For this review, take the finished solid that the model builds, in its own axes (mm). Face numbers are marked on the shaded views. Coordinates: 2 decimals unless noted, no trailing zeros. Order: outer loops, then holes, each group sorted by start corner. A loop starts at its lowest first (then second) coordinate and runs counter-clockwise, first axis right, second up. Notation, with made-up numbers: (10, 67.25) -> (57, 67.25) arc R26 cw to (57, 98.25) -> close; hole circle Ø6 at (66.25, 15). An arc over 180 degrees is marked (long way). Answer as a JSON object with one key per item and string values. Group by question number.
1) Add section D-D, the plane z = 9.5. Write out the cut boundary in (x, y), then the cut area to 3 significant figures.
2) Wall thickness on L1, parallel to X at y = 5, z = 5; L2, parallel to X at y = -17, z = 2; L3, parallel to Y at x = -13, z = 2: over which ranges is each line inside the solid? List them lowest first.
3) Add section A-A, the plane y = 0. Write out the cut boundary in (x, z).
4) Add section C-C, the plane y = -21. Write out the cut boundary in (x, z), then the cut area to 3 significant figures.
5) For pin 1 (18.5 mm diameter, centred on x = -12.51, y = 13.19, fed in from +Z); pin 2 (8 mm diameter, centred on x = -23, z = 7.5, fed in from -Y); pin 3 (12 mm diameter, centred on x = -12.5, y = -20.5, fed in from +Z); pin 4 (1 mm diameter, centred on x = 21, z = 3.5, fed in from +Y), all flat-tipped, find the tip position at first contact; note any pin that passes through.
6) Draft analysis for pull direction X (two halves, no side actions). For the marked faces 1, 2, 3 and 4, state which applies: +X half, -X half, draft (parallel to the pull), parting line (faces both ways), or undercut.
7) Add section B-B, the plane x = 13. Write out the cut boundary in (y, z).
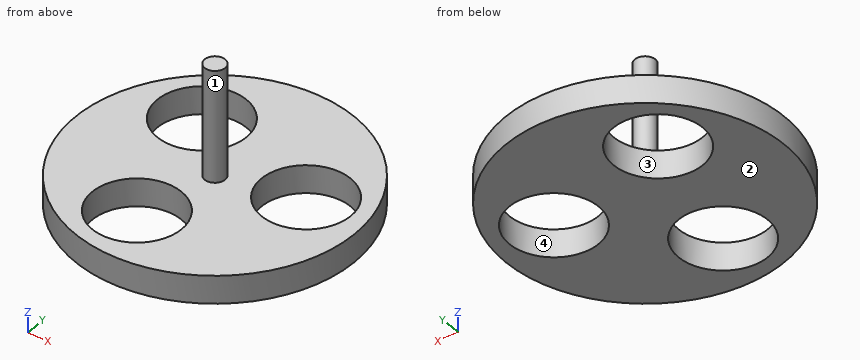
from build123d import *

# Parameters (mm, degrees)
F0_R     = 31.75
F2_DEPTH = 6.35
F1_R     = 10.16
F3_DEPTH = 25.4
F4_R     = 2.336661
F5_DEPTH = 25.4


with BuildPart() as f2:
    # F0 (on Top) → F2 (new body)
    with BuildSketch(Plane.XY):
        Circle(F0_R)
    extrude(amount=F2_DEPTH)

    # F1 (on face) → F3 (cut)
    with BuildSketch(Plane.XY):
        with Locations((-5.168118, -17.430304)):
            Circle(F1_R)
        with Locations((17.679145, 4.23943)):
            Circle(F1_R)
        with Locations((-12.511027, 13.190874)):
            Circle(F1_R)
    extrude(amount=F3_DEPTH, mode=Mode.SUBTRACT)

    # F4 (on face) → F5 (join)
    with BuildSketch(Plane.XY.offset(6.35)):
        Circle(F4_R)
    extrude(amount=F5_DEPTH)


solid = f2.part
Output values:
{
 "1": {"outline": "circle Ø4.67 at (0, 0)", "area": "17.2 mm²"},
 "2": {"L1": "x = -31.35 to -18.52, -6.5 to 7.55, 27.81 to 31.35", "L2": "x = -26.82 to -15.32, 4.98 to 26.82", "L3": "y = -28.97 to -23.9, -10.96 to 3.04, 23.34 to 28.97"},
 "3": {"outline": "(-31.75, 0) -> (8.45, 0) -> (8.45, 6.35) -> (2.34, 6.35) -> (2.34, 31.75) -> (-2.34, 31.75) -> (-2.34, 6.35) -> (-31.75, 6.35) -> close; (26.91, 0) -> (31.75, 0) -> (31.75, 6.35) -> (26.91, 6.35) -> close"},
 "4": {"outline": "(-23.81, 0) -> (-14.68, 0) -> (-14.68, 6.35) -> (-23.81, 6.35) -> close; (4.34, 0) -> (23.81, 0) -> (23.81, 6.35) -> (4.34, 6.35) -> close", "area": "182 mm²"},
 "5": {"pin 1": "passes through", "pin 2": "stops at y = -25.31", "pin 3": "stops at z = 6.35", "pin 4": "stops at y = 24.24"},
 "6": {"face 1": "parting line", "face 2": "draft", "face 3": "undercut", "face 4": "undercut"},
 "7": {"outline": "(-28.97, 0) -> (-4.78, 0) -> (-4.78, 6.35) -> (-28.97, 6.35) -> close; (13.26, 0) -> (28.97, 0) -> (28.97, 6.35) -> (13.26, 6.35) -> close"}
}
